```python
from build123d import *

# Parameters (mm, degrees)
SKETCH1_W           = 35
SKETCH1_H           = 35
SKETCH1_R           = 2
BOSS_EXTRUDE1_DEPTH = 3
SKETCH2_W           = 4
SKETCH2_H           = 35
BOSS_EXTRUDE2_DEPTH = 30
SKETCH3_R           = 4
BOSS_EXTRUDE3_DEPTH = 8


with BuildPart() as part:
    # Sketch1 → Boss-Extrude1 (new body)
    with BuildSketch(Plane(origin=(0, 0, 0), x_dir=(1, 0, 0), z_dir=(0, 1, 0))):
        Rectangle(SKETCH1_W, SKETCH1_H)
        with Locations(Location((0, 0, 0), (0, 0, 270))):
            Circle(SKETCH1_R, mode=Mode.SUBTRACT)
    extrude(amount=BOSS_EXTRUDE1_DEPTH)

    # Sketch2 → Boss-Extrude2 (add)
    with BuildSketch(Plane(origin=(0, 3, 0), x_dir=(1, 0, 0), z_dir=(0, 1, 0))):
        with Locations((-15.5, 0)):
            Rectangle(SKETCH2_W, SKETCH2_H)
    extrude(amount=BOSS_EXTRUDE2_DEPTH)

    # Sketch3 → Boss-Extrude3 (add)
    with BuildSketch(Plane.ZY.offset(17.5)):
        with Locations((0, 16.5)):
            Circle(SKETCH3_R)
    extrude(amount=BOSS_EXTRUDE3_DEPTH)


solid = part.part
```
The model under review builds one solid part; all positions refer to its coordinate system, in mm. A direction names the side the tool comes from. Give positions to 0.01 mm unless a question says otherwise; leave off trailing zeros. Write each loop counter-clockwise with the first axis right and the second up, starting at its lowest first coordinate (ties: lowest second). Pieces come first, ordered by that corner, then holes. Notation, with made-up numbers: (-4.75, -19) - (7.25, -19) arc R20 ccw to (7.25, 17) - close; hole circle Ø8 at (59.5, 69.25). An arc over 180 degrees is marked (long way). Answer in a Markdown table with one row per item. Add a question column.
1. Insertion check: P1, Ø1, axis at y = 9, z = 7.5, coming from the +X side; P2, Ø8, axis at y = 29, z = 14, coming from the -X side; P3, Ø9.5, axis at x = -5.5, z = -7, coming from the +Y side; P4, Ø3, axis at x = 0, z = 0, coming from the -Y side (3 decimals). Each pin has a flat end and moves straight along its axis. Give the tip position at first contact, or say it passes through.
2. Draft analysis for pull direction X (two halves, no side actions). For faces 1 (the cylindrical face through (-2, 1, 0)), 2 (the flat face through (-25.5, 17, 0)), 3 (the flat face through (-13.5, 18, 0)), state which applies: +X half, -X half, draft (parallel to the pull), parting line (faces both ways), or undercut.
3. Tool access review of faces 4 (the flat face through (5, 3, 0)), 5 (the flat face through (4, 0, 0)), 6 (the cylindrical face through (-21.444, 20.466, -0.521)): name each direction out of +Z, -Z, +X, -X, +Y, -Y from which nothing blocks a thin tool from reaching the whole face with its end or side.
4. We need section B-B on x = 0. Write out the cut boundary in (y, z), then the cut area to 3 significant figures.
5. Wall thickness on line 1 along X through (y, z) = (1, 0); line 2 along X through (y, z) = (28, 0); line 3 along Y through (x, z) = (-3.5, 8.5): over which ranges is each line inside the solid? List them lowest first. Write a range as [from, to].
6. We need section C-C on y = 16.5. Write out the cut boundary in (x, z).
7. We need section A-A on z = 0. Write out the cut boundary in (x, y), then the cut area to 3 significant figures.
8. We need section D-D on z = -11.5. Write out the cut boundary in (x, y), then the cut area to 3 significant figures.
Ans:
| question | item | result |
|---|---|---|
| 1 | P1 | stops at x = -13.5 |
| 1 | P2 | stops at x = -17.5 |
| 1 | P3 | stops at y = 3 |
| 1 | P4 | passes through |
| 2 | face 1 | undercut |
| 2 | face 2 | -X half |
| 2 | face 3 | +X half |
| 3 | face 4 | +Z, -Z, +X, +Y |
| 3 | face 5 | +Z, -Z, +X, -X, -Y |
| 3 | face 6 | -X |
| 4 | outline | (0, -17.5) - (3, -17.5) - (3, -2) - (0, -2) - close; (0, 2) - (3, 2) - (3, 17.5) - (0, 17.5) - close |
| 4 | area | 93.0 mm^2 |
| 5 | line 1 | x = [-17.5, -2], [2, 17.5] |
| 5 | line 2 | x = [-17.5, -13.5] |
| 5 | line 3 | y = [0, 3] |
| 6 | outline | (-25.5, -4) - (-17.5, -4) - (-17.5, -17.5) - (-13.5, -17.5) - (-13.5, 17.5) - (-17.5, 17.5) - (-17.5, 4) - (-25.5, 4) - close |
| 7 | outline | (-25.5, 12.5) - (-17.5, 12.5) - (-17.5, 0) - (-2, 0) - (-2, 3) - (-13.5, 3) - (-13.5, 33) - (-17.5, 33) - (-17.5, 20.5) - (-25.5, 20.5) - close; (2, 0) - (17.5, 0) - (17.5, 3) - (2, 3) - close |
| 7 | area | 277 mm^2 |
| 8 | outline | (-17.5, 0) - (17.5, 0) - (17.5, 3) - (-13.5, 3) - (-13.5, 33) - (-17.5, 33) - close |
| 8 | area | 225 mm^2 |
